```python
from build123d import *

# Parameters (mm, degrees)
F0_R     = 2.25
F1_DEPTH = 5
F2_DEPTH = 7.5
F4_W     = 2.75
F4_H     = 5


with BuildPart() as f1:
    # F0 (on Right) → F1 (new body)
    with BuildSketch(Plane.YZ):
        with BuildLine():
            Line((-32.5, -33.3578620553), (-32.5, 43.1248188402))
            ThreePointArc((-32.5, 43.1248188402), (-38.2073481766, 38.1601696185), (-43.1649418054, 32.4466916485))
            ThreePointArc((-43.1649418054, 32.4466916485), (-54, 0), (-43.1649418054, -32.4466916485))
            ThreePointArc((-43.1649418054, -32.4466916485), (-38.1837661841, -38.1837661841), (-32.4466916485, -43.1649418054))
            ThreePointArc((-32.4466916485, -43.1649418054), (0, -54), (32.4466916485, -43.1649418054))
            ThreePointArc((32.4466916485, -43.1649418054), (38.1837661841, -38.1837661841), (43.1649418054, -32.4466916485))
            ThreePointArc((43.1649418054, -32.4466916485), (51.2196586161, -17.1039928453), (54, 0))
            ThreePointArc((54, 0), (51.2196586161, 17.1039928453), (43.1649418054, 32.4466916485))
            ThreePointArc((43.1649418054, 32.4466916485), (38.2073481766, 38.1601696185), (32.5, 43.1248188402))
            Line((32.5, 43.1248188402), (32.5, -33.3578620553))
            ThreePointArc((32.5, -33.3578620553), (29.5710678119, -40.4289298672), (22.5, -43.3578620553))
            Line((22.5, -43.3578620553), (-22.5, -43.3578620553))
            ThreePointArc((-22.5, -43.3578620553), (-29.5710678119, -40.4289298672), (-32.5, -33.3578620553))
        make_face()
        with BuildLine():
            ThreePointArc((-32.5, 43.1248188402), (-32.4733520211, 43.1448885561), (-32.4466916485, 43.1649418054))
            ThreePointArc((-32.4466916485, 43.1649418054), (-34.4603348429, 42.5704269643), (-36.3706059725, 43.4416737844))
            Line((-36.3706059725, 43.4416737844), (-37.4644660941, 44.5355339059))
            ThreePointArc((-37.4644660941, 44.5355339059), (-44.5355339059, 44.5355339059), (-44.5355339059, 37.4644660941))
            Line((-44.5355339059, 37.4644660941), (-43.4416737844, 36.3706059725))
            ThreePointArc((-43.4416737844, 36.3706059725), (-42.5704269643, 34.4603348429), (-43.1649418054, 32.4466916485))
            ThreePointArc((-43.1649418054, 32.4466916485), (-38.2073481766, 38.1601696185), (-32.5, 43.1248188402))
        make_face()
        with Locations((-41, 41)):
            Circle(F0_R, mode=Mode.SUBTRACT)
        with BuildLine():
            ThreePointArc((32.4466916485, 43.1649418054), (32.4733520211, 43.1448885561), (32.5, 43.1248188402))
            ThreePointArc((32.5, 43.1248188402), (38.2073481766, 38.1601696185), (43.1649418054, 32.4466916485))
            ThreePointArc((43.1649418054, 32.4466916485), (42.5704269643, 34.4603348429), (43.4416737844, 36.3706059725))
            Line((43.4416737844, 36.3706059725), (44.5355339059, 37.4644660941))
            ThreePointArc((44.5355339059, 37.4644660941), (44.5355339059, 44.5355339059), (37.4644660941, 44.5355339059))
            Line((37.4644660941, 44.5355339059), (36.3706059725, 43.4416737844))
            ThreePointArc((36.3706059725, 43.4416737844), (34.4603348429, 42.5704269643), (32.4466916485, 43.1649418054))
        make_face()
        with Locations((41, 41)):
            Circle(F0_R, mode=Mode.SUBTRACT)
        with BuildLine():
            ThreePointArc((43.1649418054, -32.4466916485), (38.1837661841, -38.1837661841), (32.4466916485, -43.1649418054))
            ThreePointArc((32.4466916485, -43.1649418054), (34.4603348429, -42.5704269643), (36.3706059725, -43.4416737844))
            Line((36.3706059725, -43.4416737844), (37.4644660941, -44.5355339059))
            ThreePointArc((37.4644660941, -44.5355339059), (44.5355339059, -44.5355339059), (44.5355339059, -37.4644660941))
            Line((44.5355339059, -37.4644660941), (43.4416737844, -36.3706059725))
            ThreePointArc((43.4416737844, -36.3706059725), (42.5704269643, -34.4603348429), (43.1649418054, -32.4466916485))
        make_face()
        with Locations((41, -41)):
            Circle(F0_R, mode=Mode.SUBTRACT)
        with BuildLine():
            ThreePointArc((-32.4466916485, -43.1649418054), (-38.1837661841, -38.1837661841), (-43.1649418054, -32.4466916485))
            ThreePointArc((-43.1649418054, -32.4466916485), (-42.5704269643, -34.4603348429), (-43.4416737844, -36.3706059725))
            Line((-43.4416737844, -36.3706059725), (-44.5355339059, -37.4644660941))
            ThreePointArc((-44.5355339059, -37.4644660941), (-44.5355339059, -44.5355339059), (-37.4644660941, -44.5355339059))
            Line((-37.4644660941, -44.5355339059), (-36.3706059725, -43.4416737844))
            ThreePointArc((-36.3706059725, -43.4416737844), (-34.4603348429, -42.5704269643), (-32.4466916485, -43.1649418054))
        make_face()
        with Locations((-41, -41)):
            Circle(F0_R, mode=Mode.SUBTRACT)
    extrude(amount=F1_DEPTH)

    # F0 (on Right) → F2 (join)
    with BuildSketch(Plane.YZ):
        with BuildLine():
            ThreePointArc((-27.5, 46.4731105049), (-30.0189515962, 44.8872202867), (-32.4466916485, 43.1649418054))
            ThreePointArc((-32.4466916485, 43.1649418054), (-32.4733520211, 43.1448885561), (-32.5, 43.1248188402))
            Line((-32.5, 43.1248188402), (-32.5, -33.3578620553))
            ThreePointArc((-32.5, -33.3578620553), (-29.5710678119, -40.4289298672), (-22.5, -43.3578620553))
            Line((-22.5, -43.3578620553), (22.5, -43.3578620553))
            ThreePointArc((22.5, -43.3578620553), (29.5710678119, -40.4289298672), (32.5, -33.3578620553))
            Line((32.5, -33.3578620553), (32.5, 43.1248188402))
            ThreePointArc((32.5, 43.1248188402), (32.4733520211, 43.1448885561), (32.4466916485, 43.1649418054))
            ThreePointArc((32.4466916485, 43.1649418054), (30.0189515962, 44.8872202867), (27.5, 46.4731105049))
            Line((27.5, 46.4731105049), (27.5, -33.3578620553))
            ThreePointArc((27.5, -33.3578620553), (26.0355339059, -36.8933959612), (22.5, -38.3578620553))
            Line((22.5, -38.3578620553), (-22.5, -38.3578620553))
            ThreePointArc((-22.5, -38.3578620553), (-26.0355339059, -36.8933959612), (-27.5, -33.3578620553))
            Line((-27.5, -33.3578620553), (-27.5, 46.4731105049))
        make_face()
    extrude(amount=F2_DEPTH)

    # F5: sweep along a path in F0
    with BuildLine(Plane.YZ) as f5_path:
        Line((-27.5, 46.4731105049), (-27.5, -33.3578620553))
        ThreePointArc((-27.5, -33.3578620553), (-26.0355339059, -36.8933959612), (-22.5, -38.3578620553))
        Line((-22.5, -38.3578620553), (22.5, -38.3578620553))
        ThreePointArc((22.5, -38.3578620553), (26.0355339059, -36.8933959612), (27.5, -33.3578620553))
        Line((27.5, -33.3578620553), (27.5, 46.4731105049))
    # F4 (on plane+point) → F5 (sweep, cut)
    with BuildSketch(Plane.XY.offset(46.4731105049)):
        with Locations((3.75, -28)):
            Rectangle(F4_W, F4_H)
    sweep(path=f5_path.line, mode=Mode.SUBTRACT)


solid = f1.part
```
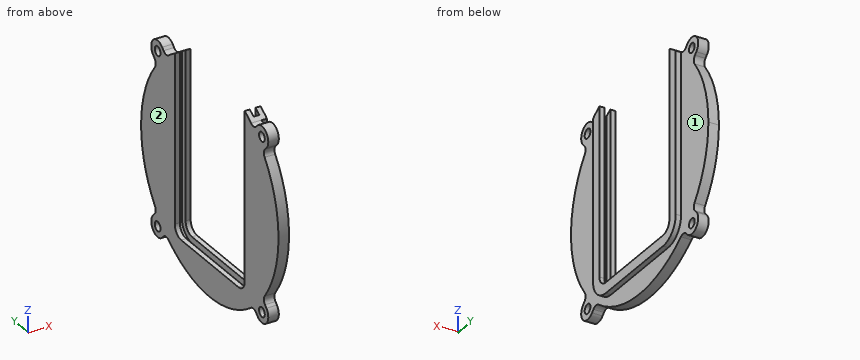
Read the model definition and answer for the solid it produces. Units are mm, in the model's axes. Face numbers are marked on the shaded views. A direction names the side the tool comes from. Round coordinates to 2 decimals unless told otherwise and drop trailing zeros. Write each loop counter-clockwise with the first axis right and the second up, starting at its lowest first coordinate (ties: lowest second). Pieces come first, ordered by that corner, then holes. Notation, with made-up numbers: (-10.75, -3) - (18.25, -3) arc R27 cw to (18.25, 19) - close; hole circle Ø5 at (-36.5, -23.5). An arc over 180 degrees is marked (long way). One line per item, written item: value.
Q1. Find section D-D (y = 29). Determine the outline of the cut face in (x, z) (3 decimals).
The answers:
outline: (0, -45.552) - (5, -45.552) - (5, -40.957) - (7.5, -40.957) - (7.5, 45.552) - (5.125, 45.552) - (5.125, -38.022) - (2.375, -38.022) - (2.375, 45.552) - (0, 45.552) - close
Q2. Straight lines are drawn through the part: line 1 (Z direction, x = 1.9, y = -41); line 2 (Y direction, x = 6.25, z = 36.5); line 3 (Y direction, x = 1.5, z = -1). For each, find the intervals that lie inside material, in ascending order. Write a range as from..to.
The answers:
line 1: z = -46..-43.25, -38.75..38.75, 43.25..46
line 2: y = -32.5..-27.5, 27.5..32.5
line 3: y = -53.99..-27.5, 27.5..53.99
Q3. Which of the six approach directions +Z, -Z, +X, -X, +Y, -Y give full straight-line access (tool end or side, diameter ignored) to the marked faces 1 and 2?
The answers:
face 1: -Z, +X
face 2: +Z, -Z, -X, +Y, -Y
Q4. Find section A-A (y = -41). Determine the outline of the cut face in (x, z).
The answers:
outline: (0, -46) - (5, -46) - (5, -43.25) - (0, -43.25) - close; (0, -38.75) - (5, -38.75) - (5, 38.75) - (0, 38.75) - close; (0, 43.25) - (5, 43.25) - (5, 46) - (0, 46) - close
Q5. Find section B-B (z = 41). Determine the outline of the cut face in (x, y) (3 decimals).
The answers:
outline: (0, -46) - (5, -46) - (5, -43.25) - (0, -43.25) - close; (0, -38.75) - (5, -38.75) - (5, -32.5) - (7.5, -32.5) - (7.5, -27.5) - (5.125, -27.5) - (5.125, -30.5) - (2.375, -30.5) - (2.375, -27.5) - (0, -27.5) - close; (0, 27.5) - (2.375, 27.5) - (2.375, 30.5) - (5.125, 30.5) - (5.125, 27.5) - (7.5, 27.5) - (7.5, 32.5) - (5, 32.5) - (5, 38.75) - (0, 38.75) - close; (0, 43.25) - (5, 43.25) - (5, 46) - (0, 46) - close
Q6. Find section C-C (z = -29). Determine the outline of the cut face in (x, y) (3 decimals), and give its area (3 significant figures).
The answers:
outline: (0, -45.552) - (5, -45.552) - (5, -32.5) - (7.5, -32.5) - (7.5, -27.5) - (5.125, -27.5) - (5.125, -30.5) - (2.375, -30.5) - (2.375, -27.5) - (0, -27.5) - close; (0, 27.5) - (2.375, 27.5) - (2.375, 30.5) - (5.125, 30.5) - (5.125, 27.5) - (7.5, 27.5) - (7.5, 32.5) - (5, 32.5) - (5, 45.552) - (0, 45.552) - close
area: 189 mm2
Q7. Each of these flat-tipped pins is pushed along its axis until it touches: P1, Ø5, axis at y = 41, z = -41, coming from the -X side; P2, Ø1.2, axis at x = 6, y = 10, coming from the -Z side; P3, Ø2.5, axis at x = 6.5, z = -8.5, coming from the -Y side; P4, Ø6, axis at y = -41, z = 41, coming from the +X side. Where does it stop, or does it pass through?
The answers:
P1: stops at x = 0
P2: stops at z = -43.36
P3: stops at y = -32.5
P4: stops at x = 5
